Autodesk Inventor part; units mm, degrees
ref_plane "YZ Plane" through (0, 0, 0) normal (1, 0, 0) x (0, 1, 0)
ref_plane "XZ Plane" through (0, 0, 0) normal (0, 1, 0) x (-1, 0, 0)
ref_plane "XY Plane" through (0, 0, 0) normal (0, 0, 1) x (1, 0, 0)
sketch "Sketch1" plane through (0, 0, 0) normal (0, 0, 1) x (1, 0, 0)
  line L0 (11.375, -6.1) -> (-11.375, -6.1)
  line L1 (-11.375, -6.1) -> (-11.375, 6.1)
  line L2 (-11.375, 6.1) -> (11.375, 6.1)
  line L3 (11.375, 6.1) -> (11.375, -6.1)
  line L4 (11.375, -6.1) -> (-11.375, 6.1) construction
  line L5 (-11.375, -6.1) -> (11.375, 6.1) construction
  point P0 (0, 0)
  dimension "d0" = 12.2
  dimension "d1" = 22.75
extrude "Extrusion1" add sketch "Sketch1" along normal blind 5.3
fillet "Fillet1" radius 0.5 4 edges at (-11.375, 6.1, 2.65) (-11.375, -6.1, 2.65) (11.375, -6.1, 2.65) (11.375, 6.1, 2.65)
fillet "Fillet1" radius 0.25 4 edges at (0, -6.1, 0) (-11.375, 0, 0) (0, 6.1, 0) (11.375, 0, 0)
sketch "Sketch2" plane through (0, 0, 5.3) normal (0, 0, 1) x (1, 0, 0)
  line L0 (10.375, -5) -> (-10.375, -5)
  line L1 (-10.375, -5) -> (-10.375, 5)
  line L2 (-10.375, 5) -> (10.375, 5)
  line L3 (10.375, 5) -> (10.375, -5)
  line L4 (10.375, -5) -> (-10.375, 5) construction
  line L5 (-10.375, -5) -> (10.375, 5) construction
  line L6 (10.875, 6.1) -> (-10.875, 6.1)
  line L7 (-11.375, 5.6) -> (-11.375, -5.6)
  line L8 (-11.375, -5.6) -> (-11.375, 5.6)
  line L9 (-10.375, -1.75) -> (-11.375, -1.75)
  line L10 (-11.375, -1.75) -> (-11.375, 1.75)
  line L11 (-11.375, 1.75) -> (-10.375, 1.75)
  line L12 (-10.375, 1.75) -> (-10.375, -1.75)
  line L13 (10, -4.5) -> (-10, -4.5) construction
  line L14 (-10, -4.5) -> (-10, 4.5) construction
  line L15 (-10, 4.5) -> (10, 4.5) construction
  line L16 (10, 4.5) -> (10, -4.5) construction
  line L17 (10, -4.5) -> (-10, 4.5) construction
  line L18 (-10, -4.5) -> (10, 4.5) construction
  circle A0 centre (-10, 4.5) radius 0.5
  circle A1 centre (10, 4.5) radius 0.5
  circle A2 centre (-10, -4.5) radius 0.5
  circle A3 centre (10, -4.5) radius 0.5
  circle A4 centre (-10, 4.5) radius 1
  circle A5 centre (10, 4.5) radius 1
  circle A6 centre (-10, -4.5) radius 1
  circle A7 centre (10, -4.5) radius 1
  point P0 (0, 0)
  point P1 (-11.375, 0)
  point P2 (0, 0)
  point P3 (-11.375, 0)
  point P4 (0, 0)
  dimension "d6" = 1.1
  dimension "d7" = 1
  dimension "d8" = 3.5
  dimension "d9" = 20
  dimension "d10" = 9
  dimension "d11" = 1
  dimension "d12" = 2
extrude "Extrusion2" cut sketch "Sketch2" against normal blind 4.5 contours L0 A3 L3 | L0 A7 L3 A3 | A3 L3 | L0 A6 L1 A4 L2 A5 L3 A7 | L0 A2 L1 A6 | L0 L1 A2 | A2 L1 | A5 L2 A1 L3 | A1 L3 | A1 L2 L3 | A4 L1 A0 L2 | A0 L1 L2 | A0 L1 picked at (10.2274, -3.7042) picked at (10.11, -4.5904) picked at (-9.1814, -4.3794) picked at (-10.0833, -4.5) picked at (10.2274, 3.7042) picked at (10.1829, 4.6853) picked at (-9.1814, 4.3794) picked at (-10.0875, 4.5371)
extrude "Extrusion3" cut sketch "Sketch2" against normal through all contours A3 L3 | L3 A3 | A2 L1 | A2 L1 | A1 L3 | L3 A1 | A0 L1 | A0 L1
extrude "Extrusion4" add sketch "Sketch2" along normal blind 2 from surface at -4.5 contours A6 L1 A2 L0 | L0 A2 L1 A6 | L0 L1 A2 | A4 L1 A0 L2 | L2 L1 A0 A4 | A0 L1 L2
extrude "Extrusion5" cut sketch "Sketch2" against normal up to surface (2.5 mm away) contours A6 L1 A2 L0 | L0 A2 L1 A6 | L0 L1 A2 | A4 L1 A0 L2 | L2 L1 A0 A4 | A0 L1 L2
extrude "Extrusion6" add sketch "Sketch2" along normal blind 3.5 from surface at -4.5 contours L3 A3 A7 L0 | L0 A3 L3 | L0 A7 L3 A3 | A5 L2 A1 L3 | L3 A1 L2 A5 | A1 L2 L3
extrude "Extrusion7" cut sketch "Sketch2" against normal up to surface (1 mm away) contours L3 A3 A7 L0 | L0 A3 L3 | L0 A7 L3 A3 | A5 L2 A1 L3 | L3 A1 L2 A5 | A1 L2 L3
extrude "Extrusion8" cut sketch "Sketch2" against normal blind 1.5 contours L9 L7 L11 L1
extrude "Extrusion9" cut sketch "Sketch2" along normal blind 0.75 from surface at -5.3 contours L3 A3 A7 L0 | L0 A3 L3 | L0 A7 L3 A3 | A6 L1 A2 L0 | L0 A2 L1 A6 | L0 L1 A2 | A5 L2 A1 L3 | L3 A1 L2 A5 | A1 L2 L3 | A4 L1 A0 L2 | L2 L1 A0 A4 | A0 L1 L2
properties part number "sevo onder" material "Glass"
Read the model definition and answer for the solid it produces. Units are mm, in the model's axes. A direction names the side the tool comes from. Round coordinates to 2 decimals unless told otherwise and drop trailing zeros. Write each loop counter-clockwise with the first axis right and the second up, starting at its lowest first coordinate (ties: lowest second). Pieces come first, ordered by that corner, then holes. Notation, with made-up numbers: M 89.5,4.5 L 143.5,4.5 A20 cw 143.5,29.5 Z; hole C -5,81.25 d7. An arc over 180 degrees is marked long. Use a Markdown table: item, result.
1) The part is cut by section C-C (z = 3.1). Write down the section's boundary in (x, y) (3 decimals), plus the area to 3 significant figures.
Answers follow:
| item | result |
|---|---|
| outline | M -11.375,-5.6 A0.5 ccw -10.875,-6.1 L 10.875,-6.1 A0.5 ccw 11.375,-5.6 L 11.375,5.6 A0.5 ccw 10.875,6.1 L -10.875,6.1 A0.5 ccw -11.375,5.6 Z; hole M -10.375,-3.573 A1 ccw long -9.134,-5 L 9.134,-5 A1 cw 10.375,-3.573 L 10.375,3.573 A1 cw 9.134,5 L -9.134,5 A1 ccw long -10.375,3.573 Z; hole C 10,-4.5 d1; hole C 10,4.5 d1 |
| area | 69.3 mm2 |
2) For a pull along Y with two mould halves and no side action, classify faces 4 (the flat face through (0, -6.1, 3)), 5 (the flat face through (0, 0, 0)), 6 (the flat face through (0, 5, 3)) as pulls with the +Y half, pulls with the -Y half, needs draft (parallel to the pull), parting line crosses it, or undercut.
Answers follow:
| item | result |
|---|---|
| face 4 | pulls with the -Y half |
| face 5 | needs draft |
| face 6 | undercut |
3) Straight lines are drawn through the part: line 1 along Y through (x, z) = (-10, 0.45); line 2 along X through (y, z) = (-4.5, 3.4) (3 decimals); line 3 along X through (y, z) = (-4.5, 0.55) (3 decimals). For each, find the intervals that lie inside material, in ascending order. Write a range as [from, to].
Answers follow:
| item | result |
|---|---|
| line 1 | y = [-6.1, -5.5], [-3.5, 3.5], [5.5, 6.1] |
| line 2 | x = [-11.375, -11], [9, 9.5], [10.5, 11.375] |
| line 3 | x = [-11.375, -11], [-9, 9], [11, 11.375] |
4) The part is cut by section A-A (x = 10). Give the number of separate pieces and of enclosed holes in the cut face, plus the area to 3 significant figures.
Answers follow:
| item | result |
|---|---|
| separate pieces | 3 |
| enclosed holes | 0 |
| area | 19.0 mm2 |
5) A tool of negligible diameter and unlimited length cuts with its end or side. For faces 1 (the cylindrical face through (9.263, 3.824, 0.37)), 2 (the flat face through (-10.375, 0, 3)), 3 (the cylindrical face through (10, 5, 3)), from which of +Z, -Z, +X, -X, +Y, -Y can it reach the whole face along a straight path? Write none if from no direction.
Answers follow:
| item | result |
|---|---|
| face 1 | -Z |
| face 2 | +Z |
| face 3 | +Z, -Z |
6) The part is cut by section D-D (y = -3.25). Write down the section's boundary in (x, z) (3 decimals), plus the area to 3 significant figures.
Answers follow:
| item | result |
|---|---|
| outline | M -11.375,0.25 A0.25 ccw -11.125,0 L 11.125,0 A0.25 ccw 11.375,0.25 L 11.375,5.3 L 10.375,5.3 L 10.375,0.8 L -10.375,0.8 L -10.375,5.3 L -11.375,5.3 Z |
| area | 27.2 mm2 |
7) Flat-ended cylindrical pins translate along their axes: pin 1 (3 mm diameter, centred on x = -5, y = 1, fed in from +Z); pin 2 (0.5 mm diameter, centred on x = -11, y = 0, fed in from +Z). Find the tip coordinate at first contact, or state that the pin passes through.
Answers follow:
| item | result |
|---|---|
| pin 1 | stops at z = 0.8 |
| pin 2 | stops at z = 3.8 |
